```python
from build123d import *

# Parameters (mm, degrees)
F1_DEPTH = 63.5
F2_DEPTH = 25.4
F3_DEPTH = 25.4
F4_DEPTH = 7.9375
F6_R     = 10.16


with BuildPart() as f1:
    # F0 (on Front) → F1 (new body, symmetric)
    with BuildSketch(Plane.XZ):
        Polygon((22.225, 9.525), (-41.275, 9.525), (-41.275, -9.525), (41.275, -9.525), (41.275, 9.525), align=None)
    extrude(amount=F1_DEPTH, both=True)

    # F0 (on Front) → F2 (join, symmetric)
    with BuildSketch(Plane.XZ):
        with BuildLine():
            Line((22.225, 27.466178), (22.225, 9.525))
            Line((22.225, 9.525), (41.275, 9.525))
            Line((41.275, 9.525), (41.275, 27.466178))
            ThreePointArc((41.275, 27.466178), (47.109768, 39.762901), (60.325, 43.020438))
            Line((60.325, 43.020438), (60.325, 62.246561))
            ThreePointArc((60.325, 62.246561), (33.60357, 53.26), (22.225, 27.466178))
        make_face()
    extrude(amount=F2_DEPTH, both=True)

    # F0 (on Front) → F3 (join, symmetric)
    with BuildSketch(Plane.XZ):
        with BuildLine():
            ThreePointArc((62.836075, 61.9252), (61.58345, 62.10864), (60.325, 62.246561))
            Line((60.325, 62.246561), (60.325, 43.020438))
            ThreePointArc((60.325, 43.020438), (60.64729, 42.951158), (60.968073, 42.8752))
            Line((60.968073, 42.8752), (83.748926, 42.8752))
            Line((83.748926, 42.8752), (83.748926, 61.9252))
            Line((83.748926, 61.9252), (62.836075, 61.9252))
        make_face()
    extrude(amount=F3_DEPTH, both=True)

    # F0 (on Front) → F4 (join, symmetric)
    with BuildSketch(Plane.XZ):
        with BuildLine():
            add(Edge.make_bspline(
                [(-41.275, 9.525), (-7.276739, 26.636683), (20.247733, 69.46599), (60.325, 62.428354)],
                knots=[0, 0, 0, 0, 114.185038, 114.185038, 114.185038, 114.185038], degree=3))
            Line((-41.275, 9.525), (22.225, 9.525))
            Line((22.225, 9.525), (22.225, 27.466178))
            ThreePointArc((22.225, 27.466178), (33.60357, 53.26), (60.325, 62.246561))
            Line((60.325, 62.246561), (60.325, 62.428354))
        make_face()
    extrude(amount=F4_DEPTH, both=True)

    # F0 (on Front) → F5 (revolve)
    with BuildSketch(Plane.XZ):
        Polygon((111.125, 66.675), (83.748926, 66.675), (83.748926, 61.9252), (83.748926, 42.8752), (83.748926, 38.1), (111.125, 38.1), align=None)
    revolve(axis=Axis((83.748926, 0, 52.3875), (0, 0, 1)))

    # F6
    f6_edges = [f1.edges().sort_by_distance(p)[0] for p in [
        (41.275, 63.5, 0),
        (-41.275, 63.5, 0),
        (41.275, -63.5, 0),
        (-41.275, -63.5, 0),
    ]]
    fillet(f6_edges, radius=F6_R)


solid = f1.part
```
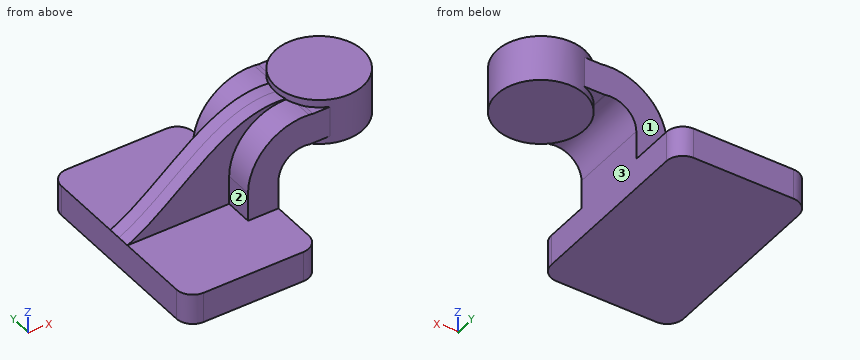
Source: CAD feature listing. Evaluate the final solid. Frame: model axes, mm. Face numbers are marked on the shaded views. A direction names the side the tool comes from. Coordinates: 2 decimals unless noted, no trailing zeros. Order: outer loops, then holes, each group sorted by start corner. A loop starts at its lowest first (then second) coordinate and runs counter-clockwise, first axis right, second up. Notation, with made-up numbers: M 54,28.25 L 69,28.25 A10 ccw 69,35.25 Z; hole C -12.5,35.5 d5. An arc over 180 degrees is marked long. Write each question's results on one line, items separated by ' | '. Start each with the question number.
1) Section query B-B (y = 34.5). Return the cut outline in (x, z) (3 decimals), plus the area to 3 significant figures.
2) Section query A-A (z = 4). Return the cut outline in (x, y) (3 decimals), plus the area to 3 significant figures.
3) Line query: line 1 (Y direction, x = -12, z = 10); line 2 (Y direction, x = 31, z = 50.5); line 3 (Z direction, x = -29.5, y = -13.5) (3 decimals). Output: solid intervals per line, ascending. Write a range as from..to.
4) Access query for the marked faces 1, 2 and 3. Directions: +Z, -Z, +X, -X, +Y, -Y. A direction counts if a zero-diameter tool reaches every point of the face in a straight line with its end or side. Return the directions, or none.
5) Contact query for flat-ended pins moving along their axis: pin 1 Ø8 at (x, y) = (68, -22) entering from -Z; pin 2 Ø6 at (y, z) = (24, 23.5) entering from -X (3 decimals); pin 3 Ø3 at (x, y) = (46, 20) entering from -Z; pin 4 Ø8 at (x, z) = (77, 32.5) entering from -Y. Output: stop coordinate, or through.
6) Section query C-C (x = 76). Return the cut outline in (y, z) (1 decimal).
Answers:
1) outline: M -41.275,-9.525 L 41.275,-9.525 L 41.275,9.525 L -41.275,9.525 Z | area: 1,570 mm^2
2) outline: M -41.275,-53.34 A10.16 ccw -31.115,-63.5 L 31.115,-63.5 A10.16 ccw 41.275,-53.34 L 41.275,53.34 A10.16 ccw 31.115,63.5 L -31.115,63.5 A10.16 ccw -41.275,53.34 Z | area: 10,400 mm^2
3) line 1: y = -7.94..7.94 | line 2: y = -25.4..25.4 | line 3: z = -9.525..9.525
4) face 1: +Z, -X, +Y | face 2: +Z, -X, -Y | face 3: -Z, +X, +Y, -Y
5) pin 1: stops at z = 38.1 | pin 2: stops at x = 22.225 | pin 3: stops at z = 37.06 | pin 4: passes through
6) outline: M -26.3,38.1 L 26.3,38.1 L 26.3,66.7 L -26.3,66.7 Z
